from build123d import *

# Parameters (mm, degrees)
SKETCH1_W                      = 19
SKETCH1_H                      = 10.7
BOSS_EXTRUDE1_DEPTH            = 38
SKETCH1_H_2                    = 2.3
BOSS_EXTRUDE1_2_DEPTH          = 38
SKETCH1_6_W                    = 12.45
SKETCH1_6_H                    = 3.2
BOSS_EXTRUDE6_DEPTH            = 38
BOSS_EXTRUDE7_DEPTH            = 16
SKETCH4_W                      = 38
SKETCH4_H                      = 2.3
SKETCH4_H_2                    = 10.7
BOSS_EXTRUDE8_DEPTH            = 3
CUT_EXTRUDE1_REACH             = 48.286
SKETCH6_R                      = 1.5
CUT_EXTRUDE1_DIRECTION_2_REACH = 48.286
BOSS_EXTRUDE10_REACH           = 45.922
SKETCH7_W                      = 2
SKETCH7_H                      = 38
BOSS_EXTRUDE11_REACH           = 46.087
SKETCH8_W                      = 7.5
SKETCH8_H                      = 38
CUT_EXTRUDE2_REACH             = 55.44
SKETCH9_R                      = 1.5
CUT_EXTRUDE3_START             = -2
SKETCH9_3_R                    = 2.9
SKETCH9_3_R_2                  = 1.5
CUT_EXTRUDE3_DEPTH             = 8.45
SKETCH6_3_R                    = 5.5
SKETCH6_3_R_2                  = 1.5
SKETCH6_3_W                    = 9.18298076
SKETCH6_3_H                    = 14.3
CUT_EXTRUDE4_DEPTH             = 7


with BuildPart() as part:
    # Sketch1 → Boss-Extrude1 (new body)
    with BuildSketch(Plane.XY):
        with Locations((7.125, 9.65)):
            Rectangle(SKETCH1_W, SKETCH1_H)
    extrude(amount=-BOSS_EXTRUDE1_DEPTH)



with BuildPart() as body_2:
    # Sketch1 → Boss-Extrude1 2 (new body)
    with BuildSketch(Plane.XY):
        with Locations((7.125, -3.85)):
            Rectangle(SKETCH1_W, SKETCH1_H_2)
    extrude(amount=-BOSS_EXTRUDE1_2_DEPTH)


with BuildPart() as part_1:
    add(part.part)

    add(body_2.part)  # Boss-Extrude6 merges body 2
    # Sketch1<6> → Boss-Extrude6 (add)
    with BuildSketch(Plane.XY):
        Polygon((-14.825, 5), (-14.825, -2), (-9.825, -2), (-9.825, -5), (-2.375, -5), (-2.375, 5), align=None)
        with Locations((-8.6, 13.4)):
            Rectangle(SKETCH1_6_W, SKETCH1_6_H)
    extrude(amount=-BOSS_EXTRUDE6_DEPTH)

    # Sketch1<7> → Boss-Extrude7 (add)
    with BuildSketch(Plane.XY):
        Polygon((-14.825, -2), (-14.825, -3.3), (-14.825, -5), (-9.825, -5), (-9.825, -2), align=None)
    extrude(amount=-BOSS_EXTRUDE7_DEPTH)

    # Sketch4 → Boss-Extrude8 (add)
    with BuildSketch(Plane(origin=(16.625, 0, 0), x_dir=(0, 0, -1), z_dir=(1, 0, 0))):
        with Locations((19, -3.85)):
            Rectangle(SKETCH4_W, SKETCH4_H)
        with Locations((19, 9.65)):
            Rectangle(SKETCH4_W, SKETCH4_H_2)
    extrude(amount=BOSS_EXTRUDE8_DEPTH)

    # Sketch6 → Cut-Extrude1 (cut, up to next)
    with BuildSketch(Plane(origin=(0, -2.7, 0), x_dir=(1, 0, 0), z_dir=(0, 1, 0)), mode=Mode.PRIVATE) as cut_extrude1_sk1:
        with Locations(Location((10.44201924, 23.7, 0), (0, 0, 270))):
            Circle(SKETCH6_R)
    cut_extrude1_tool1 = extrude(cut_extrude1_sk1.sketch, amount=-CUT_EXTRUDE1_REACH, mode=Mode.PRIVATE) & part_1.part
    # Sketch6 → Cut-Extrude1 (cut, up to next)
    with BuildSketch(Plane(origin=(0, -2.7, 0), x_dir=(1, 0, 0), z_dir=(0, 1, 0)), mode=Mode.PRIVATE) as cut_extrude1_sk2:
        with BuildLine():
            Line((10.44201924, 25.2), (10.44201924, 23.7))
            Line((10.44201924, 23.7), (11.94201924, 23.7))
            ThreePointArc((11.94201924, 23.7), (11.502679412, 24.760660172), (10.44201924, 25.2))
        make_face()
    cut_extrude1_tool2 = extrude(cut_extrude1_sk2.sketch, amount=-CUT_EXTRUDE1_REACH, mode=Mode.PRIVATE) & part_1.part
    # Sketch6 → Cut-Extrude1 (cut, up to next)
    with BuildSketch(Plane(origin=(0, -2.7, 0), x_dir=(1, 0, 0), z_dir=(0, 1, 0)), mode=Mode.PRIVATE) as cut_extrude1_sk3:
        with BuildLine():
            Line((11.94201924, 23.7), (10.44201924, 23.7))
            Line((10.44201924, 23.7), (10.44201924, 25.2))
            ThreePointArc((10.44201924, 25.2), (9.381359068, 22.639339828), (11.94201924, 23.7))
        make_face()
    cut_extrude1_tool3 = extrude(cut_extrude1_sk3.sketch, amount=-CUT_EXTRUDE1_REACH, mode=Mode.PRIVATE) & part_1.part
    add(cut_extrude1_tool1.solids().sort_by_distance((10.442019, -2.7, -23.7))[0], mode=Mode.SUBTRACT)
    add(cut_extrude1_tool2.solids().sort_by_distance((11.078639, -2.7, -24.33662))[0], mode=Mode.SUBTRACT)
    add(cut_extrude1_tool3.solids().sort_by_distance((10.229813, -2.7, -23.487793))[0], mode=Mode.SUBTRACT)

    # Cut-Extrude1 direction 2: up to this face of the body (flat: up to its plane)
    cut_extrude1_direction_2_end = Plane(part_1.part.faces().sort_by_distance((2.4, 15, -19))[0])
    # Sketch6 → Cut-Extrude1 direction 2 (cut, up to the picked face)
    with BuildSketch(Plane(origin=(0, -2.7, 0), x_dir=(1, 0, 0), z_dir=(0, 1, 0)), mode=Mode.PRIVATE) as cut_extrude1_direction_2_sk1:
        with Locations(Location((10.44201924, 23.7, 0), (0, 0, 270))):
            Circle(SKETCH6_R)
    cut_extrude1_direction_2_tool1 = split(extrude(cut_extrude1_direction_2_sk1.sketch, amount=CUT_EXTRUDE1_DIRECTION_2_REACH, mode=Mode.PRIVATE), bisect_by=cut_extrude1_direction_2_end, keep=Keep.BOTH, mode=Mode.PRIVATE)
    # Sketch6 → Cut-Extrude1 direction 2 (cut, up to the picked face)
    with BuildSketch(Plane(origin=(0, -2.7, 0), x_dir=(1, 0, 0), z_dir=(0, 1, 0)), mode=Mode.PRIVATE) as cut_extrude1_direction_2_sk2:
        with BuildLine():
            Line((10.44201924, 25.2), (10.44201924, 23.7))
            Line((10.44201924, 23.7), (11.94201924, 23.7))
            ThreePointArc((11.94201924, 23.7), (11.502679412, 24.760660172), (10.44201924, 25.2))
        make_face()
    cut_extrude1_direction_2_tool2 = split(extrude(cut_extrude1_direction_2_sk2.sketch, amount=CUT_EXTRUDE1_DIRECTION_2_REACH, mode=Mode.PRIVATE), bisect_by=cut_extrude1_direction_2_end, keep=Keep.BOTH, mode=Mode.PRIVATE)
    # Sketch6 → Cut-Extrude1 direction 2 (cut, up to the picked face)
    with BuildSketch(Plane(origin=(0, -2.7, 0), x_dir=(1, 0, 0), z_dir=(0, 1, 0)), mode=Mode.PRIVATE) as cut_extrude1_direction_2_sk3:
        with BuildLine():
            Line((11.94201924, 23.7), (10.44201924, 23.7))
            Line((10.44201924, 23.7), (10.44201924, 25.2))
            ThreePointArc((10.44201924, 25.2), (9.381359068, 22.639339828), (11.94201924, 23.7))
        make_face()
    cut_extrude1_direction_2_tool3 = split(extrude(cut_extrude1_direction_2_sk3.sketch, amount=CUT_EXTRUDE1_DIRECTION_2_REACH, mode=Mode.PRIVATE), bisect_by=cut_extrude1_direction_2_end, keep=Keep.BOTH, mode=Mode.PRIVATE)
    add(cut_extrude1_direction_2_tool1.solids().sort_by(Axis((10.442019, -2.7, -23.7), (0, 1, 0)))[0], mode=Mode.SUBTRACT)
    add(cut_extrude1_direction_2_tool2.solids().sort_by(Axis((11.078639, -2.7, -24.33662), (0, 1, 0)))[0], mode=Mode.SUBTRACT)
    add(cut_extrude1_direction_2_tool3.solids().sort_by(Axis((10.229813, -2.7, -23.487793), (0, 1, 0)))[0], mode=Mode.SUBTRACT)

    # Sketch7 → Boss-Extrude10 (add, up to next)
    with BuildSketch(Plane(origin=(0, 5, 0), x_dir=(1, 0, 0), z_dir=(0, 1, 0)), mode=Mode.PRIVATE) as boss_extrude10_sk1:
        with Locations((-3.375, 19)):
            Rectangle(SKETCH7_W, SKETCH7_H)
    boss_extrude10_tool1 = extrude(boss_extrude10_sk1.sketch, amount=BOSS_EXTRUDE10_REACH, mode=Mode.PRIVATE) - part_1.part
    # Sketch7 → Boss-Extrude10 (add, up to next)
    with BuildSketch(Plane(origin=(0, 5, 0), x_dir=(1, 0, 0), z_dir=(0, 1, 0)), mode=Mode.PRIVATE) as boss_extrude10_sk2:
        with Locations((-13.825, 19)):
            Rectangle(SKETCH7_W, SKETCH7_H)
    boss_extrude10_tool2 = extrude(boss_extrude10_sk2.sketch, amount=BOSS_EXTRUDE10_REACH, mode=Mode.PRIVATE) - part_1.part
    add(boss_extrude10_tool1.solids().sort_by_distance((-3.375, 5, -19))[0])
    add(boss_extrude10_tool2.solids().sort_by_distance((-13.825, 5, -19))[0])

    # Sketch8 → Boss-Extrude11 (add, up to next)
    with BuildSketch(Plane.XZ.offset(-4.3), mode=Mode.PRIVATE) as boss_extrude11_sk1:
        with Locations((15.875, -19)):
            Rectangle(SKETCH8_W, SKETCH8_H)
    boss_extrude11_tool1 = extrude(boss_extrude11_sk1.sketch, amount=BOSS_EXTRUDE11_REACH, mode=Mode.PRIVATE) - part_1.part
    add(boss_extrude11_tool1.solids().sort_by_distance((15.875, 4.3, -19))[0])

    # Sketch9 → Cut-Extrude2 (cut, up to next)
    with BuildSketch(Plane.ZY.offset(14.825), mode=Mode.PRIVATE) as cut_extrude2_sk1:
        with Locations(Location((-5.5, 6.75, 0), (0, 0, 270))):
            Circle(SKETCH9_R)
    cut_extrude2_tool1 = extrude(cut_extrude2_sk1.sketch, amount=-CUT_EXTRUDE2_REACH, mode=Mode.PRIVATE) & part_1.part
    add(cut_extrude2_tool1.solids().sort_by_distance((-14.825, 6.75, -5.5))[0], mode=Mode.SUBTRACT)

    # Sketch9<3> → Cut-Extrude3 (cut)
    with BuildSketch(Plane.ZY.offset(14.825).offset(CUT_EXTRUDE3_START)):
        with Locations((-5.5, 6.75)):
            Circle(SKETCH9_3_R)
        with Locations(Location((-5.5, 6.75, 0), (0, 0, 270))):
            Circle(SKETCH9_3_R_2, mode=Mode.SUBTRACT)
    extrude(amount=-CUT_EXTRUDE3_DEPTH, mode=Mode.SUBTRACT)

    # Sketch6<3> → Cut-Extrude4 (cut)
    with BuildSketch(Plane(origin=(0, -2.7, 0), x_dir=(1, 0, 0), z_dir=(0, 1, 0))):
        with Locations((10.44201924, 23.7)):
            Circle(SKETCH6_3_R)
        with Locations(Location((10.44201924, 23.7, 0), (0, 0, 270))):
            Circle(SKETCH6_3_R_2, mode=Mode.SUBTRACT)
        with Locations((15.03350962, 30.85)):
            Rectangle(SKETCH6_3_W, SKETCH6_3_H)
    extrude(amount=CUT_EXTRUDE4_DEPTH, mode=Mode.SUBTRACT)


with BuildPart() as body_2_2:
    # Mirror2: mirrored copy
    add(part_1.part.mirror(Plane.XY))


solid = body_2_2.part
Check sheet for the modelled part. Datum: model origin and axes. Units: mm. A direction names the side the tool comes from. Give positions to 0.01 mm unless a question says otherwise; leave off trailing zeros. Write each loop counter-clockwise with the first axis right and the second up, starting at its lowest first coordinate (ties: lowest second). Pieces come first, ordered by that corner, then holes. Notation, with made-up numbers: (17.5, 35) -> (39.5, 35) arc R6 cw to (39.5, 43) -> close; hole circle Ø4 at (-38, -26.5). An arc over 180 degrees is marked (long way). One line per item, written item: value. Start each with the question number.
Item 1: Draft check along X on faces 6 (the flat face through (18, 1, 23.7)), 7 (the flat face through (19.625, 5, 19)), 8 (the cylindrical face through (11.93, 9.58, 23.9)). Enter one of: +X half, -X half, draft (parallel to the pull), parting line (faces both ways), or undercut.
Item 2: Gauge pin test, flat ends, axial feed: pin 1 (2.5 mm diameter, centred on x = -12.5, y = -3.5, fed in from +Z); pin 2 (2.5 mm diameter, centred on y = -4, z = 22.5, fed in from -X) (3 decimals); pin 3 (1.5 mm diameter, centred on x = -11.5, z = 28.5, fed in from -Y). Record the tip position at first contact, or that the pin passes through.
Item 3: Section check A-A on y = 10.5. Record the cut outline in (x, z) (3 decimals).
Item 4: Material ranges on probe 1 along Y at (x, z) = (11.5, 32); probe 2 along Y at (x, z) = (-5.5, 25); probe 3 along Z at (x, y) = (-13.3, 6.75), recorded low to high. Write a range as from..to.
Item 5: Tool access check on faces 1 (the cylindrical face through (14.858, 0.751, 20.421)), 2 (the flat face through (2, 7, 38)), 3 (the flat face through (-14.825, 5, 19)), 4 (the flat face through (-2.375, 1, 19)), 5 (the flat face through (-9.825, -3, 27)). Record the directions out of +Z, -Z, +X, -X, +Y, -Y that give a thin tool (end or side, any length) a straight path to the whole face; none if there is none.
Item 6: Section check D-D on z = 5.5. Record the cut outline in (x, y) (3 decimals), then the cut area to 3 significant figures.
Item 7: Section check B-B on x = -8.5. Record the cut outline in (y, z).
Item 8: Section check C-C on y = 2.5. Record the cut outline in (x, z) (3 decimals), then the cut area to 3 significant figures.
Results list:
1. face 6: draft
1. face 7: +X half
1. face 8: undercut
2. pin 1: z = 16
2. pin 2: x = -9.825
2. pin 3: y = -2
3. outline: (-14.825, 0) -> (-12.825, 0) -> (-12.825, 38) -> (-14.825, 38) -> close; (-4.375, 0) -> (19.625, 0) -> (19.625, 38) -> (-4.375, 38) -> close; hole circle Ø3 at (10.442, 23.7)
4. probe 1: -5..-2.7, 4.3..15
4. probe 2: -5..5, 11.8..15
4. probe 3: 0..4, 7..38
5. face 1: +Z
5. face 2: +Z, +X, -X, +Y, -Y
5. face 3: +Z, -Z, -X, +Y, -Y
5. face 4: +Z, -Z
5. face 5: +Z, -X, -Y
6. outline: (-14.825, -5) -> (19.625, -5) -> (19.625, 15) -> (-14.825, 15) -> (-14.825, 8.25) -> (-12.825, 8.25) -> (-12.825, 11.8) -> (-4.375, 11.8) -> (-4.375, 3.85) -> (-12.825, 3.85) -> (-12.825, 5.25) -> (-14.825, 5.25) -> close; hole (-2.375, -2.7) -> (12.125, -2.7) -> (12.125, 4.3) -> (-2.375, 4.3) -> close
6. area: 514 mm²
7. outline: (-5, 0) -> (5, 0) -> (5, 3.19) arc R2.9 cw to (5, 7.81) -> (5, 38) -> (-5, 38) -> close; (11.8, 0) -> (15, 0) -> (15, 38) -> (11.8, 38) -> close
8. outline: (-14.825, 0) -> (-2.375, 0) -> (-2.375, 38) -> (-14.825, 38) -> close; (12.125, 0) -> (19.625, 0) -> (19.625, 23.7) -> (15.942, 23.7) arc R5.5 cw to (12.125, 18.464) -> close
8. area: 636 mm²
